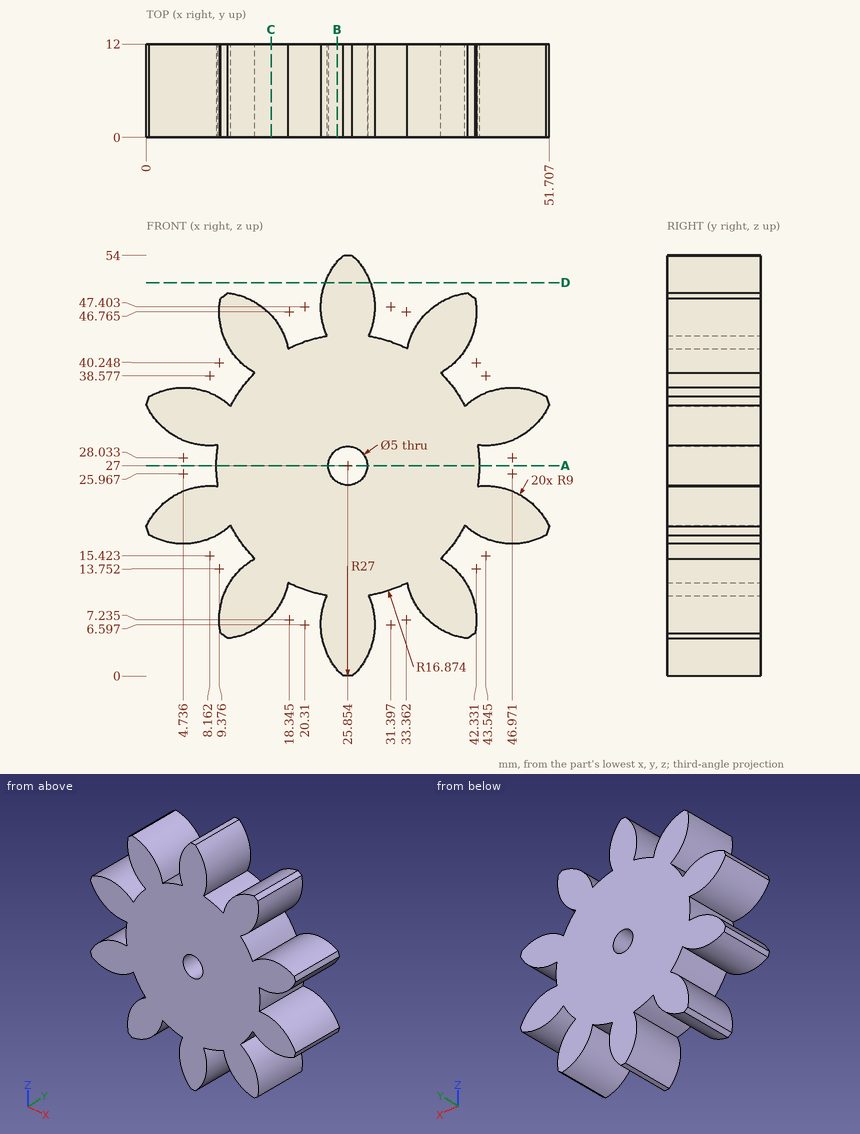
Job drawing, mm, ordinate dimensions from the low corner. One solid piece. Coordinates: 2 decimals unless noted, no trailing zeros. Order: outer loops, then holes, each group sorted by start corner. A loop starts at its lowest first (then second) coordinate and runs counter-clockwise, first axis right, second up. Notation, with made-up numbers: (38, 51.25) - (74, 51.25) arc R21 ccw to (74, 78.25) - close; hole circle Ø9 at (4.25, -5.75). An arc over 180 degrees is marked (long way). Write each question's results on one line, items separated by ' | '. Start each with the question number.
Item 1: Flat gauge pins, fed straight in: pin 1 (3 mm diameter, centred on x = 41, y = 4, fed in from -Z); pin 2 (2 mm diameter, centred on x = 5.5, y = 5, fed in from -Z). Where does each tip first touch, or does it go through?
Item 2: Band-saw the part on A-A on z = 27. Write the cut outline in (x, y).
Item 3: Band-saw the part on D-D on z = 50.5. Write the cut outline in (x, y).
Item 4: Band-saw the part on B-B on x = 24.5. Write the cut outline in (y, z) (1 decimal).
Item 5: Band-saw the part on C-C on x = 16. Write the cut outline in (y, z).
Item 6: Wall check: probe 1 along X at (y, z) = (6.5, 27); probe 2 along Z at (x, y) = (13, 8.5) (1 decimal); probe 3 along Z at (x, y) = (10.5, 9.5) (1 decimal). Give the ranges that are in metal, low to high. Write a range as [from, to].
Numbers:
1) pin 1: z = 4.82 | pin 2: z = 16.97
2) outline: (8.98, 0) - (23.35, 0) - (23.35, 12) - (8.98, 12) - close; (28.35, 0) - (42.73, 0) - (42.73, 12) - (28.35, 12) - close
3) outline: (22.95, 0) - (28.76, 0) - (28.76, 12) - (22.95, 12) - close
4) outline: (0, 0.8) - (12, 0.8) - (12, 24.9) - (0, 24.9) - close; (0, 29.1) - (12, 29.1) - (12, 53.2) - (0, 53.2) - close
5) outline: (0, 7.66) - (12, 7.66) - (12, 46.34) - (0, 46.34) - close
6) probe 1: [8.98, 23.35], [28.35, 42.73] | probe 2: [5.5, 14.5], [16.1, 37.9], [39.5, 48.5] | probe 3: [4.8, 11.6], [19.1, 34.9], [42.4, 49.2]
